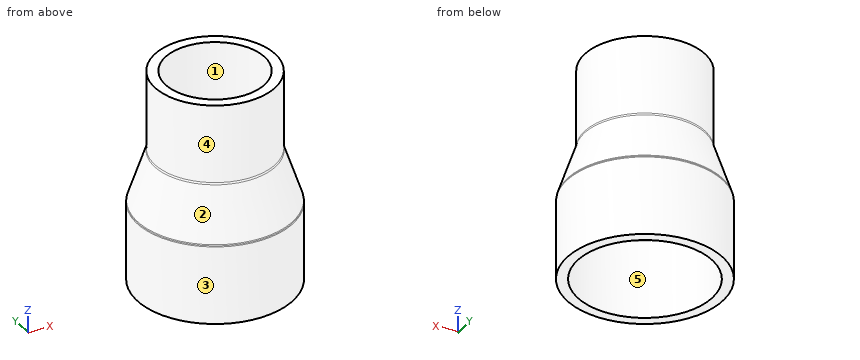
from build123d import *


with BuildPart() as f1:
    # F0 (on Front) → F1 (revolve)
    with BuildSketch(Plane.XZ):
        with BuildLine():
            Line((28.956, 50.8), (23.876, 50.8))
            Line((23.876, 50.8), (23.876, 13.217675))
            ThreePointArc((23.876, 13.217675), (23.88664, 12.957967), (23.918487, 12.7))
            ThreePointArc((23.918487, 12.7), (23.969673, 12.452136), (24.040439, 12.209137))
            Line((24.040439, 12.209137), (32.220561, -12.209137))
            ThreePointArc((32.220561, -12.209137), (32.343621, -12.706747), (32.385, -13.217675))
            Line((32.385, -13.217675), (32.385, -50.8))
            Line((32.385, -50.8), (37.465, -50.8))
            Line((37.465, -50.8), (37.465, -13.217675))
            ThreePointArc((37.465, -13.217675), (37.45436, -12.957967), (37.422513, -12.7))
            ThreePointArc((37.422513, -12.7), (37.371327, -12.452136), (37.300561, -12.209137))
            Line((37.300561, -12.209137), (29.120439, 12.209137))
            ThreePointArc((29.120439, 12.209137), (28.997379, 12.706747), (28.956, 13.217675))
            Line((28.956, 13.217675), (28.956, 50.8))
        make_face()
    revolve(axis=Axis((0, 0, 0), (0, 0, -1)))


solid = f1.part
Part model, mm, in its own coordinate system. Face numbers are marked on the shaded views. A direction names the side the tool comes from. Give positions to 0.01 mm unless a question says otherwise; leave off trailing zeros. Loops run counter-clockwise (first coordinate to the right, second up) from the corner with the lowest first, then second, coordinate; pieces in that order, holes last. Notation, with made-up numbers: (34, 48.5) -> (64, 48.5) arc R21 ccw to (64, 68.5) -> close; hole circle Ø7 at (24, -12.5). An arc over 180 degrees is marked (long way). Write each question's results on one line, items separated by ' | '. Start each with the question number.
Q1. Pull direction X, two halves, no side cores. Call the marked faces 1 and 2: +X half, -X half, draft (parallel to the pull), parting line (faces both ways), or undercut.
Q2. Pin check, flat tips, straight feed: P1, Ø1.5, axis at x = -19, z = 8.5, coming from the -Y side; P2, Ø8, axis at x = -26, z = 40.5, coming from the +Y side; P3, Ø1.5, axis at x = 27, z = 35, coming from the +Y side; P4, Ø12, axis at x = 0, y = 12.5, coming from the -Z side. Stop position of each tip, or through.
Q3. Band-saw the part on C-C on z = 16.5. List the corners of the cut face in (x, y), plus the area to 3 significant figures.
Q4. Band-saw the part on A-A on x = 0. List the corners of the cut face in (y, z) (3 decimals).
Q5. Band-saw the part on D-D on z = -25. List the corners of the cut face in (x, y) (3 decimals), plus the area to 3 significant figures.
Q6. Wall check: L1, parallel to Y at x = 0, z = 28; L2, parallel to Y at x = 0, z = -34 (3 decimals). Give the ranges that are in metal, low to high.
Q7. Which spindle directions (+Z, -Z, +X, -X, +Y, -Y) get a long thin tool onto all of the face, cutting with end or side? Do the marked faces 3, 4 and 5. Say none if no direction does.
Results are:
1) face 1: undercut | face 2: parting line
2) P1: stops at y = -24.35 | P2: stops at y = 18.83 | P3: stops at y = 12.22 | P4: passes through
3) outline: circle Ø57.91 at (0, 0); hole circle Ø47.75 at (0, 0) | area: 843 mm²
4) outline: (-37.465, -50.8) -> (-32.385, -50.8) -> (-32.385, -13.218) arc R3.175 cw to (-32.221, -12.209) -> (-24.04, 12.209) arc R3.175 ccw to (-23.918, 12.7) arc R3.175 ccw to (-23.876, 13.218) -> (-23.876, 50.8) -> (-28.956, 50.8) -> (-28.956, 13.218) arc R3.175 cw to (-29.12, 12.209) -> (-37.301, -12.209) arc R3.175 ccw to (-37.423, -12.7) arc R3.175 ccw to (-37.465, -13.218) -> close; (23.876, 13.218) arc R3.175 ccw to (23.918, 12.7) arc R3.175 ccw to (24.04, 12.209) -> (32.221, -12.209) arc R3.175 cw to (32.385, -13.218) -> (32.385, -50.8) -> (37.465, -50.8) -> (37.465, -13.218) arc R3.175 ccw to (37.423, -12.7) arc R3.175 ccw to (37.301, -12.209) -> (29.12, 12.209) arc R3.175 cw to (28.956, 13.218) -> (28.956, 50.8) -> (23.876, 50.8) -> close
5) outline: circle Ø74.93 at (0, 0); hole circle Ø64.77 at (0, 0) | area: 1,110 mm²
6) L1: y = -28.96 to -23.88, 23.88 to 28.96 | L2: y = -37.465 to -32.385, 32.385 to 37.465
7) face 3: +Z, -Z | face 4: +Z | face 5: -Z
